Model file for the job. Use its own axes, mm. Face numbers are marked on the shaded views. Round coordinates to 2 decimals unless told otherwise and drop trailing zeros. Order: outer loops, then holes, each group sorted by start corner. A loop starts at its lowest first (then second) coordinate and runs counter-clockwise, first axis right, second up. Notation, with made-up numbers: M -35.5,59.5 L -26.5,59.5 A6 ccw -26.5,66.5 Z; hole C 5.25,27.5 d11. An arc over 180 degrees is marked long. Return JSON: item names as keys, results as strings. Group by question number.
Item 1: Probe line 1 along X through (y, z) = (7.5, -74); line 2 along X through (y, z) = (5.25, -158); line 3 along Y through (x, z) = (96.5, 31). List the from-to ranges inside material, lowest first.
Item 2: Slice it at B-B on y = 16. Give the number of separate pieces and of enclosed holes in the cut face, then the cut area to 3 significant figures.
Item 3: Pin check, flat tips, straight feed: pin 1 Ø3 at (y, z) = (1.5, -165.5) entering from -X; pin 2 Ø1 at (y, z) = (8.5, -48.5) entering from -X; pin 3 Ø3 at (y, z) = (12, -11) entering from -X. Stop position of each tip, or through.
Item 4: Slice it at A-A on x = -4. Write the cut outline in (y, z), then the cut area to 3 significant figures.
Item 5: Pull direction Z, two halves, no side cores. Call the marked faces 1 and 2: pulls with the +Z half, pulls with the -Z half, needs draft (parallel to the pull), parting line crosses it, or undercut.
from build123d import *

# Parameters (mm, degrees)
SKETCH1_R         = 130.175
EXTRUDE1_DEPTH    = 6.35
SKETCH3_R         = 4.7625
EXTRUDE3_DEPTH    = 6.35
SKETCH2_R         = 3.175
EXTRUDE4_DEPTH    = 12.7
CIRPATTERN1_COUNT = 48
EXTRUDE5_DEPTH    = 19.05
CIRPATTERN2_COUNT = 5


with BuildPart() as part:
    # Sketch1 → Extrude1 (new body)
    with BuildSketch(Plane(origin=(0, 0, 0), x_dir=(1, 0, 0), z_dir=(0, 1, 0))):
        with Locations(Location((19.489328739, 73.663551537, 0), (0, 0, 270))):  # turned: the seam where the file's is
            Circle(SKETCH1_R)
    extrude(amount=EXTRUDE1_DEPTH)

    # Sketch3 → Extrude3 (cut)
    with BuildSketch(Plane(origin=(0, 6.35, 0), x_dir=(1, 0, 0), z_dir=(0, 1, 0))):
        with Locations(Location((19.489328739, 73.663551537, 0), (0, 0, 270))):  # turned: the seam where the file's is
            Circle(SKETCH3_R)
    extrude(amount=-EXTRUDE3_DEPTH, mode=Mode.SUBTRACT)

    # Sketch2 → Extrude4 (add)
    with BuildSketch(Plane(origin=(0, 6.35, 0), x_dir=(-1, 0, 0), z_dir=(0, 1, 0))):
        with Locations(Location((-143.949328739, -73.663551537, 0), (0, 0, 90))):  # turned: the seam where the file's is
            Circle(SKETCH2_R)
    extrude4 = extrude(amount=EXTRUDE4_DEPTH)

    # CirPattern1: Extrude4 ×48 about axis
    cirpattern1_axis = Axis((19.489328739, 0, -73.663551537), (0, 1, 0))
    for i in range(1, CIRPATTERN1_COUNT):
        add(extrude4.rotate(cirpattern1_axis, i * 360 / CIRPATTERN1_COUNT))

    # Sketch5 → Extrude5 (cut)
    with BuildSketch(Plane(origin=(0, 6.35, 0), x_dir=(1, 0, 0), z_dir=(0, 1, 0))):
        with BuildLine():
            Line((-16.382042301, 109.534922577), (-61.369324084, 154.52220436))
            ThreePointArc((-61.369324084, 154.52220436), (-24.271058832, 179.310472705), (19.489328739, 188.014954995))
            Line((19.489328739, 188.014954995), (19.489328739, 124.393330962))
            ThreePointArc((19.489328739, 124.393330962), (0.075882625, 120.531756437), (-16.382042301, 109.534922577))
        make_face()
    extrude5 = extrude(amount=-EXTRUDE5_DEPTH, mode=Mode.SUBTRACT)

    # CirPattern2: Extrude5 ×5 about axis
    cirpattern2_axis = Axis((19.489328739, 0, -73.663551537), (0, 1, 0))
    for i in range(1, CIRPATTERN2_COUNT):
        add(extrude5.rotate(cirpattern2_axis, i * 360 / CIRPATTERN2_COUNT), mode=Mode.SUBTRACT)


solid = part.part
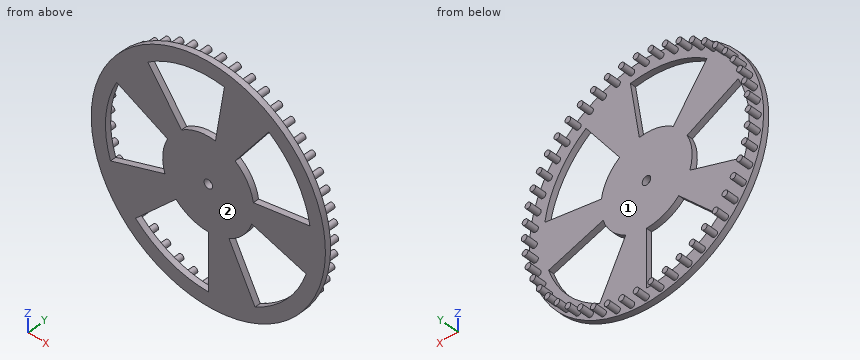
Output values:
{
 "1": {"line 1": "-108.13 to -101.81, 140.79 to 147.11", "line 2": "-79.67 to -57.74, 19.49 to 62.46, 96.71 to 118.65", "line 3": "0 to 6.35"},
 "2": {"separate pieces": "48", "enclosed holes": "0", "area": "1,520 mm²"},
 "3": {"pin 1": "x = -74.24", "pin 2": "through", "pin 3": "x = -91.47"},
 "4": {"outline": "M 0,-201.7 L 6.35,-201.7 L 6.35,-185.58 L 0,-185.58 Z; M 0,-118.63 L 6.35,-118.63 L 6.35,-28.7 L 0,-28.7 Z; M 0,38.25 L 6.35,38.25 L 6.35,54.37 L 0,54.37 Z", "area": "776 mm²"},
 "5": {"face 1": "undercut", "face 2": "needs draft"}
}
